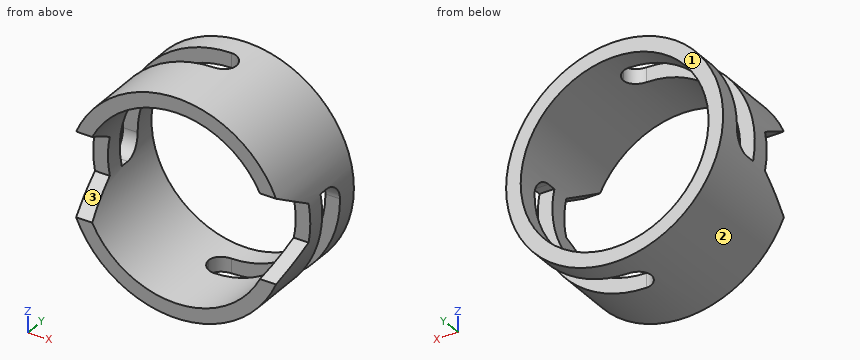
```python
from build123d import *

# Parameters (mm, degrees)
F0_R          = 70.65
F1_DEPTH      = 70
F2_T          = -9.5
F4_DEPTH      = 70.651
F4_DEPTH_BACK = 70.651
F6_DEPTH      = 70.6510001
F8_DEPTH      = 70.6510001


with BuildPart() as f1:
    # F0 (on Front) → F1 (new body)
    with BuildSketch(Plane.XZ):
        Circle(F0_R)
    extrude(amount=F1_DEPTH)

    # F2
    f2_openings = [f1.faces().sort_by_distance(p)[0] for p in [
        (0, -70, 0),
        (0, 0, 0),
    ]]
    offset(amount=F2_T, openings=f2_openings)

    # F3 (on Right) → F4 (cut, two sides)
    with BuildSketch(Plane.YZ) as f4_sk:
        with BuildLine():
            Line((-26, 12.5), (-32, 12.5))
            Line((-32, 12.5), (-32, -12.5))
            Line((-32, -12.5), (-26, -12.5))
            ThreePointArc((-26, -12.5), (-17.5147186258, -8.9852813742), (-14, -0.5))
            Line((-14, -0.5), (-14, 0.5))
            ThreePointArc((-14, 0.5), (-17.5147186258, 8.9852813742), (-26, 12.5))
        make_face()
        Polygon((-70, 27.5), (-70, 12.5), (-70, -12.5), (-70, -27.5), (-44.0192378865, -12.5), (-44.0192378865, 12.5), align=None)
    extrude(amount=-F4_DEPTH, mode=Mode.SUBTRACT)
    extrude(f4_sk.sketch, amount=F4_DEPTH_BACK, mode=Mode.SUBTRACT)

    # F5 (on Top) → F6 (cut, through all)
    with BuildSketch(Plane.XY):
        with BuildLine():
            ThreePointArc((-8.9995123916, -23.0936841124), (-6.3307520481, -29.3969976165), (0, -32))
            Line((0, -32), (79.6814696193, -32))
            Line((79.6814696193, -32), (79.6814696193, -14))
            Line((79.6814696193, -14), (0, -14))
            ThreePointArc((0, -14), (-6.3969976165, -16.6692479519), (-8.9995123916, -23.0936841124))
        make_face()
    extrude(amount=-F6_DEPTH, mode=Mode.SUBTRACT)

    # F7 (on Top) → F8 (cut, through all)
    with BuildSketch(Plane.XY):
        with BuildLine():
            Line((-108.6236870661, -32), (0, -32))
            ThreePointArc((0, -32), (6.3639610307, -29.3639610307), (9, -23))
            ThreePointArc((9, -23), (6.3639610307, -16.6360389693), (0, -14))
            Line((0, -14), (-108.6236870661, -14))
            Line((-108.6236870661, -14), (-108.6236870661, -32))
        make_face()
    extrude(amount=F8_DEPTH, mode=Mode.SUBTRACT)


solid = f1.part
```
Geometry: final body of the model. Coordinates: model frame, mm. Face numbers are marked on the shaded views. Coordinates: 2 decimals unless noted, no trailing zeros. Order: outer loops, then holes, each group sorted by start corner. A loop starts at its lowest first (then second) coordinate and runs counter-clockwise, first axis right, second up. Notation, with made-up numbers: M 61,35 L 87,35 A14 ccw 87,42 Z; hole C -27,23.5 d3. An arc over 180 degrees is marked long. Answer in a Markdown table with one row per item. Add a question column.
Q1. Section query B-B on z = -56. Return the cut outline in (x, y), and give its area (3 significant figures).
Q2. Section query A-A on x = 43. Return the cut outline in (y, z).
Q3. Section query C-C on y = -10.5. Return the cut outline in (x, z), and give its area (3 significant figures).
Q4. Contact query for flat-ended pins moving along their axis: P1, Ø12, axis at x = -65, z = -1.5, coming from the -Y side; P2, Ø5, axis at x = 55.5, y = -62, coming from the +Z side; P3, Ø3, axis at y = -44.5, z = 4, coming from the +X side. Output: stop coordinate, or through.
Q5. Mould query, pull axis Z, two halves, no side actions, for the marked faces 1, 2 and 3. Classes: released by +Z, released by -Z, zero draft, split by the parting line, or undercut.
Q6. Line query: L1, parallel to X at y = -34.5, z = -2; L2, parallel to Z at x = 0, y = -51; L3, parallel to X at y = -11.5, z = -30.5. Output: solid intervals per line, ascending.
Completed:
| question | item | result |
|---|---|---|
| 1 | outline | M -43.07,-70 L -24.56,-70 L -24.56,0 L -43.07,0 Z; M 24.56,-70 L 43.07,-70 L 43.07,-32 L 24.56,-32 Z; M 24.56,-14 L 43.07,-14 L 43.07,0 L 24.56,0 Z |
| 1 | area | 2,260 mm2 |
| 2 | outline | M -70,-56.06 L -32,-56.06 L -32,-43.48 L -70,-43.48 Z; M -70,43.48 L 0,43.48 L 0,56.06 L -70,56.06 Z; M -14,-56.06 L 0,-56.06 L 0,-43.48 L -14,-43.48 Z |
| 3 | outline | C 0,0 d141.3; hole C 0,0 d122.3 |
| 3 | area | 3,930 mm2 |
| 4 | P1 | stops at y = -44.02 |
| 4 | P2 | stops at z = 46.72 |
| 4 | P3 | stops at x = 70.6 |
| 5 | face 1 | zero draft |
| 5 | face 2 | split by the parting line |
| 5 | face 3 | undercut |
| 6 | L1 | x = -70.62 to -61.12, 61.12 to 70.62 |
| 6 | L2 | z = -70.65 to -61.15, 61.15 to 70.65 |
| 6 | L3 | x = -63.73 to -53, 53 to 63.73 |
